```python
from build123d import *

# Parameters (mm, degrees)
F0_R     = 3.175
F1_DEPTH = 9


# Not quite as in the source:
# - ends of sketch curves that miss each other by under 0.0002 mm in the source are joined


with BuildPart() as f1:
    # F0 (on Top) → F1 (new body)
    with BuildSketch(Plane.XY):
        Polygon((10.95823, -37.5), (0, -14), (0, -37.5), align=None)
        with BuildLine():
            ThreePointArc((0, -14), (-9.8994949366, -9.8994949366), (-14, 0))
            Line((-14, 0), (-37.5, 0))
            Line((-37.5, 0), (-37.5, -29.5))
            ThreePointArc((-37.5, -29.5), (-35.1568542495, -35.1568542495), (-29.5, -37.5))
            Line((-29.5, -37.5), (0, -37.5))
            Line((0, -37.5), (0, -14))
        make_face()
        with Locations((-26.324893, -26)):
            Circle(F0_R, mode=Mode.SUBTRACT)
        with BuildLine():
            Line((37.5, 0), (14, 0))
            ThreePointArc((14, 0), (12.787539009, -5.6990215031), (9.3601648439, -10.4109228263))
            Line((9.3601648439, -10.4109228263), (21.992009, -37.5))
            Line((21.992009, -37.5), (29.5, -37.5))
            ThreePointArc((29.5, -37.5), (35.1568542495, -35.1568542495), (37.5, -29.5))
            Line((37.5, -29.5), (37.5, 0))
        make_face()
        with Locations((26.324893, -26)):
            Circle(F0_R, mode=Mode.SUBTRACT)
        with BuildLine():
            Line((29.5, 37.5), (0, 37.5))
            Line((0, 37.5), (0, 14))
            ThreePointArc((0, 14), (9.8994949366, 9.8994949366), (14, 0))
            Line((14, 0), (37.5, 0))
            Line((37.5, 0), (37.5, 29.5))
            ThreePointArc((37.5, 29.5), (35.1568542495, 35.1568542495), (29.5, 37.5))
        make_face()
        with Locations((26.324893, 26)):
            Circle(F0_R, mode=Mode.SUBTRACT)
        with BuildLine():
            Line((0, 14), (0, 37.5))
            Line((0, 37.5), (-29.5, 37.5))
            ThreePointArc((-29.5, 37.5), (-35.1568542495, 35.1568542495), (-37.5, 29.5))
            Line((-37.5, 29.5), (-37.5, 0))
            Line((-37.5, 0), (-14, 0))
            ThreePointArc((-14, 0), (-9.8994949366, 9.8994949366), (0, 14))
        make_face()
        with Locations((-26.324893, 26)):
            Circle(F0_R, mode=Mode.SUBTRACT)
    extrude(amount=F1_DEPTH)


solid = f1.part
```
For this review, take the finished solid that the model builds, in its own axes (mm). Give positions to 0.01 mm unless a question says otherwise; leave off trailing zeros. Write each loop counter-clockwise with the first axis right and the second up, starting at its lowest first coordinate (ties: lowest second). Pieces come first, ordered by that corner, then holes. Notation, with made-up numbers: M 32.25,31 L 68.25,31 A24 ccw 68.25,48 Z; hole C 38,-21.5 d8. An arc over 180 degrees is marked long. Answer as a JSON object with one key per item and string values. Group by question number.
Item 1: Draft analysis for pull direction X (two halves, no side actions). For faces 1 (the flat face through (5.556, -25.914, 4.437)), 2 (the flat face through (26, -37.5, 4)), 3 (the cylindrical face through (35.094, -35.219, 4.437)), state which applies: +X half, -X half, draft (parallel to the pull), parting line (faces both ways), or undercut.
Item 2: Consider section B-B on x = -4. Write out the cut boundary in (y, z), plus the area to 3 significant figures.
Item 3: Consider section A-A on y = 26. Write out the cut boundary in (x, z).
Item 4: For probe 1 along Y at (x, z) = (-27.5, 4); probe 2 along Y at (x, z) = (23.5, 2.75); probe 3 along X at (y, z) = (26.5, 2), list the stretches that pass through material, from the lowest coordinate up. Write a range as [from, to].
Item 5: Consider section D-D on y = -5.5. Write out the cut boundary in (x, z).
Item 6: Consider section C-C on z = 6.25. Write out the cut boundary in (x, y) (3 decimals).
Item 7: For pin 1 Ø2 at (x, y) = (17, -20.5) entering from -Z, flat-tipped, find the tip position at first contact; note if it passes through.
Check result:
{
 "1": {"face 1": "undercut", "face 2": "draft", "face 3": "+X half"},
 "2": {"outline": "M -37.5,0 L -13.42,0 L -13.42,9 L -37.5,9 Z; M 13.42,0 L 37.5,0 L 37.5,9 L 13.42,9 Z", "area": "434 mm^2"},
 "3": {"outline": "M -37.5,0 L -29.5,0 L -29.5,9 L -37.5,9 Z; M -23.15,0 L 23.15,0 L 23.15,9 L -23.15,9 Z; M 29.5,0 L 37.5,0 L 37.5,9 L 29.5,9 Z"},
 "4": {"probe 1": "y = [-37.5, -28.95], [-23.05, 23.05], [28.95, 37.5]", "probe 2": "y = [-37.5, -27.45], [-24.55, 24.55], [27.45, 37.5]", "probe 3": "x = [-37.5, -29.46], [-23.19, 23.19], [29.46, 37.5]"},
 "5": {"outline": "M -37.5,0 L -12.87,0 L -12.87,9 L -37.5,9 Z; M 12.87,0 L 37.5,0 L 37.5,9 L 12.87,9 Z"},
 "6": {"outline": "M -37.5,-29.5 A8 ccw -29.5,-37.5 L 10.958,-37.5 L 0,-14 A14 cw long 9.36,-10.411 L 21.992,-37.5 L 29.5,-37.5 A8 ccw 37.5,-29.5 L 37.5,29.5 A8 ccw 29.5,37.5 L -29.5,37.5 A8 ccw -37.5,29.5 Z; hole C -26.325,-26 d6.35; hole C -26.325,26 d6.35; hole C 26.325,-26 d6.35; hole C 26.325,26 d6.35"},
 "7": {"pin 1": "stops at z = 0"}
}
